```python
from build123d import *

# Parameters (mm, degrees)
F0_R     = 10
F1_DEPTH = 40
F2_DEPTH = 20


# Not quite as in the source:
# - ends of sketch curves that miss each other by under 0.0002 mm in the source are joined


with BuildPart() as f1:
    # F0 (on Top) → F1 (new body)
    with BuildSketch(Plane.XY):
        with BuildLine():
            ThreePointArc((-108.6277332274, -19.9999968788), (-94.4928212548, -14.1381846275), (-88.6389067712, 0))
            ThreePointArc((-88.6389067712, 0), (-94.4928212535, 14.1381846263), (-108.6277332239, 19.9999968788))
            ThreePointArc((-108.6277332239, 19.9999968788), (-128.6389067712, 1.7e-09), (-108.6277332274, -19.9999968788))
        make_face()
        with Locations((-108.6389067712, 0)):
            Circle(F0_R, mode=Mode.SUBTRACT)
    extrude(amount=F1_DEPTH)

    # F0 (on Top) → F2 (join)
    with BuildSketch(Plane.XY):
        with BuildLine():
            ThreePointArc((-108.6277332239, 19.9999968788), (-94.4928212535, 14.1381846263), (-88.6389067712, 0))
            ThreePointArc((-88.6389067712, 0), (-94.4928212548, -14.1381846275), (-108.6277332274, -19.9999968788))
            Line((-108.6277332274, -19.9999968788), (-28.6277332239, -20.0000031212))
            Line((-28.6277332239, -20.0000031212), (-28.6277332239, 19.9999968788))
            Line((-28.6277332239, 19.9999968788), (-108.6277332239, 19.9999968788))
        make_face()
    extrude(amount=F2_DEPTH)


solid = f1.part
```
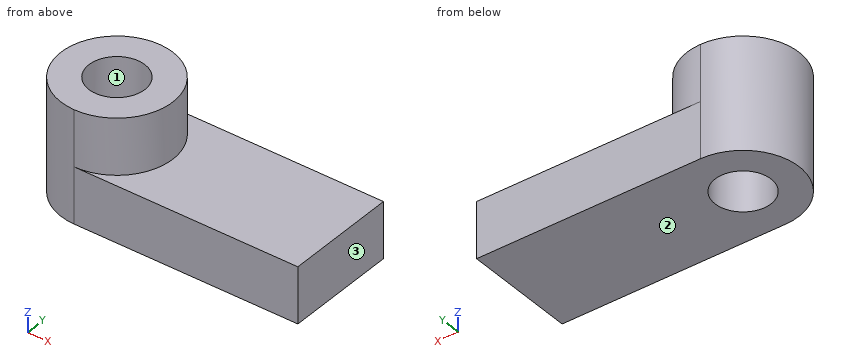
Geometry check sheet. Reference: the model listing, model coordinates, mm. Face numbers are marked on the shaded views. Coordinates: 2 decimals unless noted, no trailing zeros. Write each loop counter-clockwise with the first axis right and the second up, starting at its lowest first coordinate (ties: lowest second). Pieces come first, ordered by that corner, then holes. Notation, with made-up numbers: M 32,47.25 L 46,47.25 A26 cw 46,69.25 Z; hole C 33.25,-9 d10. An arc over 180 degrees is marked long. Answer as a JSON object with one key per item and string values.
1. Section check A-A, the plane y = 0. Enter the section's corners in (x, z), plus the area to 3 significant figures.
Answers below:
{"outline": "M -128.64,0 L -118.64,0 L -118.64,40 L -128.64,40 Z; M -98.64,0 L -28.63,0 L -28.63,20 L -88.64,20 L -88.64,40 L -98.64,40 Z", "area": "2,000 mm²"}
2. Section check B-B, the plane z = 10. Enter the section's corners in (x, y).
Answers below:
{"outline": "M -108.63,-20 L -28.63,-20 L -28.63,20 L -108.63,20 A20 ccw Z; hole C -108.64,0 d20"}
3. Section check C-C, the plane x = -103. Enter the section's corners in (y, z), plus the area to 3 significant figures.
Answers below:
{"outline": "M -20,0 L -8.26,0 L -8.26,40 L -19.19,40 L -19.19,20 L -20,20 Z; M 8.26,0 L 20,0 L 20,20 L 19.19,20 L 19.19,40 L 8.26,40 Z", "area": "907 mm²"}
4. Go/stop test with flat-tipped pins: pin 1 Ø5 at (y, z) = (-15.5, 27.5) entering from -X; pin 2 Ø20 at (x, y) = (-53.5, -7.5) entering from +Z; pin 3 Ø8 at (y, z) = (14.5, 14.5) entering from -X; pin 4 Ø3 at (x, y) = (-80.5, 11) entering from -Z. Record where each tip stops, or that it passes through.
Answers below:
{"pin 1": "stops at x = -123.84", "pin 2": "stops at z = 20", "pin 3": "stops at x = -125.66", "pin 4": "stops at z = 0"}
5. Scan lines: L1, parallel to Z at x = -51, y = -2.5; L2, parallel to Y at x = -122, z = 22; L3, parallel to X at y = -11, z = 16. Record each from-to range of solid material in increasing order.
Answers below:
{"L1": "z = 0 to 20", "L2": "y = -14.88 to 14.88", "L3": "x = -125.34 to -28.63"}
6. Draft check along X on the marked faces 1, 2 and 3. Enter one of: released by +X, released by -X, zero draft, split by the parting line, or undercut.
Answers below:
{"face 1": "undercut", "face 2": "zero draft", "face 3": "released by +X"}
7. Section check D-D, the plane y = 15. Enter the section's corners in (x, z).
Answers below:
{"outline": "M -121.87,0 L -28.63,0 L -28.63,20 L -95.41,20 L -95.41,40 L -121.87,40 Z"}
